Geometry check sheet. Reference: the model listing, model coordinates, mm. A direction names the side the tool comes from. Give positions to 0.01 mm unless a question says otherwise; leave off trailing zeros. Loops run counter-clockwise (first coordinate to the right, second up) from the corner with the lowest first, then second, coordinate; pieces in that order, holes last. Notation, with made-up numbers: (-6, 12.5) -> (24, 12.5) arc R28 cw to (24, 34.5) -> close; hole circle Ø9 at (27.5, -24). An arc over 180 degrees is marked (long way). One line per question, with ' | ' between items.
from build123d import *

# Parameters (mm, degrees)
SKETCH_W                 = 95
SKETCH_H                 = 20
PAD_DEPTH                = 20
SKETCH001_W              = 20
SKETCH001_H              = 20
SKETCH001_R              = 4
POCKET_DEPTH             = 6
SKETCH003_W              = 12
SKETCH003_H              = 11
POCKET001_DEPTH          = 2
CLONE_PLACEMENT_ANGLE    = 270
CLONE001_PLACEMENT_ANGLE = 90


with BuildPart() as part:
    # Sketch → Pad (new body)
    with BuildSketch(Plane.XY):
        Rectangle(SKETCH_W, SKETCH_H)
    extrude(amount=-PAD_DEPTH)

    # Sketch001 (on Face2 of Pad) → Pocket (cut)
    with BuildSketch(Plane.YZ.offset(47.5)):
        with Locations((0, -10)):
            Rectangle(SKETCH001_W, SKETCH001_H)
        with Locations((0, -10)):
            Circle(SKETCH001_R, mode=Mode.SUBTRACT)
    extrude(amount=-POCKET_DEPTH, mode=Mode.SUBTRACT)

    # Sketch003 (on Face2 of Pocket) → Pocket001 (cut)
    with BuildSketch(Plane.XY):
        with Locations((35.5, 0)):
            Rectangle(SKETCH003_W, SKETCH003_H)
        with Locations((-4.5, 0)):
            Rectangle(SKETCH003_W, SKETCH003_H)
    extrude(amount=-POCKET001_DEPTH, mode=Mode.SUBTRACT)


with BuildPart() as part_1:
    # Clone placement: moved
    add(part.part.moved(Location((-10, 0, -47.5))).rotate(Axis((-10, 0, -47.5), (0, 1, 0)), CLONE_PLACEMENT_ANGLE))


with BuildPart() as part_2:
    # Clone001 placement: moved
    add(part_1.part.moved(Location((6, 0, -10))).rotate(Axis((6, 0, -10), (0, 1, 0)), CLONE001_PLACEMENT_ANGLE))


solid = part_2.part
Item 1: Sectioned sample at C-C (z = -15). Record the cut outline in (x, y), plus the area to 3 significant figures.
Result:
outline: (-89, -10) -> (0, -10) -> (0, 10) -> (-89, 10) -> close | area: 1,780 mm2
Item 2: Scan lines: probe 1 along Y at (x, z) = (-40.5, -1.75); probe 2 along X at (y, z) = (4.25, -15.25); probe 3 along X at (y, z) = (3.75, -1). Record each from-to range of solid material in increasing order.
Result:
probe 1: -10 to -5.5, 5.5 to 10 | probe 2: -89 to 0 | probe 3: -89 to -52, -40 to -12
Item 3: Release check for a two-part mould opening along X. For faces 1 (the face through (-46, 0, -2)), 2 (the face through (-45, 0, -20)), 3 (the face through (0, -0.1, -14.3)), 4 (the face through (-46, -5.5, -1)) record: pulls with the +X half, pulls with the -X half, needs draft (parallel to the pull), parting line crosses it, or undercut.
Result:
face 1: undercut | face 2: needs draft | face 3: pulls with the +X half | face 4: undercut
Item 4: Sectioned sample at A-A (z = -10). Record the cut outline in (x, y), plus the area to 3 significant figures.
Result:
outline: (-89, -10) -> (0, -10) -> (0, -4) -> (6, -4) -> (6, 4) -> (0, 4) -> (0, 10) -> (-89, 10) -> close | area: 1,830 mm2
Item 5: Depth check by flat-ended pin: pin 1 Ø3.5 at (x, y) = (-45.5, 0) entering from +Z; pin 2 Ø0.6 at (y, z) = (0, -1) entering from +X; pin 3 Ø1.6 at (y, z) = (-1.5, -1.5) entering from +X; pin 4 Ø12 at (x, y) = (-4.5, -1) entering from +Z. Enter the tip coordinate at first touch or a pass-through.
Result:
pin 1: z = -2 | pin 2: x = -12 | pin 3: x = 0 | pin 4: z = 0
Item 6: Set-up check for faces 5 (the face through (-55, 0, 0)), 6 (the face through (6, 0, -10)), 7 (the face through (-52, 0, -1)), 8 (the face through (3.042, -0.867, -13.905)), 9 (the face through (-6, 0, -2)): record each of +Z, -Z, +X, -X, +Y, -Y from which the full face is reachable in a straight line by a thin tool's end or side.
Result:
face 5: +Z, +X, -X, +Y, -Y | face 6: +Z, -Z, +X, +Y, -Y | face 7: +Z | face 8: +X | face 9: +Z, +X
Item 7: Sectioned sample at B-B (y = 0). Record the cut outline in (x, z).
Result:
outline: (-89, -20) -> (0, -20) -> (0, -14) -> (6, -14) -> (6, -6) -> (0, -6) -> (0, -2) -> (-12, -2) -> (-12, 0) -> (-40, 0) -> (-40, -2) -> (-52, -2) -> (-52, 0) -> (-89, 0) -> close
